Autodesk Inventor part; units mm, degrees
ref_plane "YZ Plane" through (0, 0, 0) normal (1, 0, 0) x (0, 1, 0)
ref_plane "XZ Plane" through (0, 0, 0) normal (0, 1, 0) x (-1, 0, 0)
ref_plane "XY Plane" through (0, 0, 0) normal (0, 0, 1) x (1, 0, 0)
sketch "Sketch1" plane through (0, 0, 0) normal (0, 0, 1) x (1, 0, 0)
  line L0 (-19, 19) -> (19, 19)
  line L1 (19, 19) -> (19, -19)
  line L2 (19, -19) -> (-19, -19)
  line L3 (-19, -19) -> (-19, 19)
  line L4 (-19, 19) -> (19, -19) construction
  line L5 (19, 19) -> (-19, -19) construction
  line L6 (-11, 11) -> (11, 11)
  line L7 (11, 11) -> (11, -11)
  line L8 (11, -11) -> (-11, -11)
  line L9 (-11, -11) -> (-11, 11)
  line L10 (-11, 11) -> (11, -11) construction
  line L11 (11, 11) -> (-11, -11) construction
  point P0 (0, 0)
  dimension "d0" = 38
  dimension "d1" = 38
  dimension "d2" = 22
  dimension "d3" = 22
extrude "Extrusion1" add sketch "Sketch1" along normal mid plane 2
sketch "Sketch2" plane through (0, 0, 1) normal (0, 0, 1) x (1, 0, 0)
  line L0 (-13, 13) -> (13, 13)
  line L1 (13, 13) -> (13, -13)
  line L2 (13, -13) -> (-13, -13)
  line L3 (-13, -13) -> (-13, 13)
  line L4 (-13, 13) -> (13, -13) construction
  line L5 (13, 13) -> (-13, -13) construction
  line L6 (-11.5, -11.5) -> (11.5, -11.5)
  line L7 (11.5, -11.5) -> (11.5, 11.5)
  line L8 (11.5, 11.5) -> (-11.5, 11.5)
  line L9 (-11.5, 11.5) -> (-11.5, -11.5)
  line L10 (-11.5, -11.5) -> (11.5, 11.5) construction
  line L11 (11.5, -11.5) -> (-11.5, 11.5) construction
  point P0 (0, 0)
  dimension "d6" = 26
  dimension "d7" = 26
  dimension "d8" = 23
extrude "Extrusion2" add sketch "Sketch2" along normal blind 40
sketch "Sketch3" plane through (0, 0, -1) normal (0, 0, -1) x (-1, 0, 0)
  line L0 (11, -11) -> (11, 11)
  line L1 (11, 11) -> (-11, 11)
  line L2 (-11, 11) -> (-11, -11)
  line L3 (-11, -11) -> (11, -11)
  line L4 (19, 19) -> (19, -19)
  line L5 (19, -19) -> (-19, -19)
  line L6 (-19, -19) -> (-19, 19)
  line L7 (-19, 19) -> (19, 19)
  point P0 (0, 0)
  point P1 (15, -15)
  point P2 (-15, -15)
  point P3 (15, 15)
  point P4 (-15, 15)
  dimension "d11" = 15
  dimension "d12" = 15
  dimension "d15" = 30
  dimension "d18" = 30
hole "Hole1" at (-15, -15, -1) at (15, -15, -1) at (-15, 15, -1) at (15, 15, -1) direction (0, 0, 1) diameter 3.4 end through all
equation "\"d1\" = d0"
equation "\"d3\" = d2"
equation "\"d7\" = d6"
properties part number "pmtholder"
Verification items for the finished model (mm, model axes). A direction names the side the tool comes from. Coordinates: 2 decimals unless noted, no trailing zeros. Write each loop counter-clockwise with the first axis right and the second up, starting at its lowest first coordinate (ties: lowest second). Pieces come first, ordered by that corner, then holes. Notation, with made-up numbers: (70, 9) - (128, 9) arc R17 ccw to (128, 15) - close; hole circle Ø3 at (18, 78.25). An arc over 180 degrees is marked (long way). Answer as a JSON object with one key per item and string values.
(1) Thickness scan on line 1 along Y through (x, z) = (15, 0); line 2 along Y through (x, z) = (-7, 29.5). Record the ranges inside material, lowest first.
Report:
{"line 1": "-19 to -16.7, -13.3 to 13.3, 16.7 to 19", "line 2": "-13 to -11.5, 11.5 to 13"}
(2) Mould release check, pull along X, two halves, no side actions. Record for faces 6 (the flat face through (0, 13, 21)), 7 (the flat face through (-11.5, 0, 21)), 8 (the flat face through (13, 0, 21)): pulls with the +X half, pulls with the -X half, needs draft (parallel to the pull), parting line crosses it, or undercut.
Report:
{"face 6": "needs draft", "face 7": "undercut", "face 8": "pulls with the +X half"}
(3) Gauge pin test, flat ends, axial feed: pin 1 Ø11.5 at (x, z) = (1, 22) entering from -Y; pin 2 Ø1.5 at (x, z) = (-12.5, 12.5) entering from +Y; pin 3 Ø21 at (y, z) = (-3.5, 29) entering from +X. Record the tip position at first contact, or that the pin passes through.
Report:
{"pin 1": "y = -13", "pin 2": "y = 13", "pin 3": "x = 13"}
(4) Cross-section at C-C on x = 6.5. Record the cut outline in (y, z), plus the area to 3 significant figures.
Report:
{"outline": "(-19, -1) - (-11, -1) - (-11, 1) - (-11.5, 1) - (-11.5, 41) - (-13, 41) - (-13, 1) - (-19, 1) - close; (11, -1) - (19, -1) - (19, 1) - (13, 1) - (13, 41) - (11.5, 41) - (11.5, 1) - (11, 1) - close", "area": "152 mm^2"}
(5) Tool access check on faces 1 (the flat face through (0, 11, 0)), 2 (the flat face through (0, -13, 21)), 3 (the flat face through (-13, 0, 21)), 4 (the flat face through (0, -19, 0)), 5 (the flat face through (0, -11.5, 21)). Record the directions out of +Z, -Z, +X, -X, +Y, -Y that give a thin tool (end or side, any length) a straight path to the whole face; none if there is none.
Report:
{"face 1": "+Z, -Z", "face 2": "+Z, +X, -X, -Y", "face 3": "+Z, -X, +Y, -Y", "face 4": "+Z, -Z, +X, -X, -Y", "face 5": "+Z"}
(6) Cross-section at A-A on x = -15. Record the cut outline in (y, z).
Report:
{"outline": "(-19, -1) - (-16.7, -1) - (-16.7, 1) - (-19, 1) - close; (-13.3, -1) - (13.3, -1) - (13.3, 1) - (-13.3, 1) - close; (16.7, -1) - (19, -1) - (19, 1) - (16.7, 1) - close"}
